Read the model definition and answer for the solid it produces. Units are mm, in the model's axes. A direction names the side the tool comes from. Coordinates: 2 decimals unless noted, no trailing zeros. Write each loop counter-clockwise with the first axis right and the second up, starting at its lowest first coordinate (ties: lowest second). Pieces come first, ordered by that corner, then holes. Notation, with made-up numbers: (-34, 15) -> (-7, 15) arc R14 cw to (-7, 19) -> close; hole circle Ø3 at (49.5, 8.5). An arc over 180 degrees is marked (long way). One line per item, written item: value. Start each with the question number.
1. Consider line 1 along Z through (x, y) = (0, 18); line 2 along X through (y, z) = (-42, 8). Determine where each line is inside the solid, lowest interval first.
2. Find section C-C, the plane x = 0. Write down the section's boundary in (y, z), and give its area (3 significant figures).
3. Find section D-D, the plane x = 24.5. Write down the section's boundary in (y, z).
4. For faces 1 (the flat face through (-30, 5, 20)), 2 (the cylindrical face through (-3.905, 0.7, -29.745)), 3 (the flat face through (63.479, 4.93, 7.606)), 4 (the flat face through (24, 10, 35)), 5 (the flat face through (50, 15, 100)), determine the directions among +Z, -Z, +X, -X, +Y, -Y from which every point of the face is accessible in a straight line to the end or side of a thin tool.
5. Given P1, Ø2, axis at x = 80.5, z = 48, coming from the +Y side; P2, Ø1, axis at x = 49.5, z = 12, coming from the -Y side; P3, Ø10, axis at x = 20.5, y = -11.5, coming from the +Z side, each flat-ended and moving along its own axis, determine where each tip first touches the part or whether it passes through.
6. Find section B-B, the plane z = 84.5. Write down the section's boundary in (x, y), and give its area (3 significant figures).
7. Find section A-A, the plane y = 17.5. Write down the section's boundary in (x, z), and give its area (3 significant figures).
```python
from build123d import *

# Parameters (mm, degrees)
SKETCH1_R                = 30
SKETCH1_R_2              = 15
BOSS_EXTRUDE1_DEPTH      = 10
SKETCH1_3_R              = 30
SKETCH1_3_R_2            = 15
BOSS_EXTRUDE2_DEPTH      = 50
BOSS_EXTRUDE2_DEPTH_BACK = 50
BOSS_EXTRUDE3_DEPTH      = 30


with BuildPart() as part:
    # Sketch1 → Boss-Extrude1 (new body)
    with BuildSketch(Plane(origin=(0, 0, 0), x_dir=(1, 0, 0), z_dir=(0, 1, 0))):
        Circle(SKETCH1_R)
        Circle(SKETCH1_R_2, mode=Mode.SUBTRACT)
        with BuildLine():
            ThreePointArc((30, 0), (0, -30), (-30, 0))
            Line((-30, 0), (-30, -40))
            Line((-30, -40), (44.477364607, -115.187247331))
            ThreePointArc((44.477364607, -115.187247331), (41.7229458, -47.830649341), (108.548527268, -38.951472732))
            Line((108.548527268, -38.951472732), (17.129116361, 24.629116361))
            ThreePointArc((17.129116361, 24.629116361), (26.588282107, 13.894720385), (30, 0))
        make_face()
        with BuildLine():
            Line((110, -80), (110, -120))
            ThreePointArc((110, -120), (80, -30), (50, -120))
            Line((50, -120), (50, -80))
            ThreePointArc((50, -80), (80, -50), (110, -80))
        make_face()
    extrude(amount=BOSS_EXTRUDE1_DEPTH)

    # Sketch1_3 → Boss-Extrude2 (add, two sides)
    with BuildSketch(Plane(origin=(0, 0, 0), x_dir=(1, 0, 0), z_dir=(0, 1, 0))) as boss_extrude2_sk:
        Circle(SKETCH1_3_R)
        Circle(SKETCH1_3_R_2, mode=Mode.SUBTRACT)
    extrude(amount=BOSS_EXTRUDE2_DEPTH)
    extrude(boss_extrude2_sk.sketch, amount=-BOSS_EXTRUDE2_DEPTH_BACK)

    # Sketch1_4 → Boss-Extrude3 (add)
    with BuildSketch(Plane(origin=(0, 0, 0), x_dir=(1, 0, 0), z_dir=(0, 1, 0))):
        with BuildLine():
            Line((110, -80), (110, -120))
            ThreePointArc((110, -120), (80, -30), (50, -120))
            Line((50, -120), (50, -80))
            ThreePointArc((50, -80), (80, -50), (110, -80))
        make_face()
    extrude(amount=BOSS_EXTRUDE3_DEPTH)


solid = part.part
```
Answer block:
1. line 1: z = -30 to -15, 15 to 30
1. line 2: x = -28.91 to -12.69, 12.69 to 28.91
2. outline: (-50, -30) -> (50, -30) -> (50, -15) -> (-50, -15) -> close; (-50, 15) -> (50, 15) -> (50, 30) -> (10, 30) -> (10, 70.29) -> (0, 70.29) -> (0, 30) -> (-50, 30) -> close
2. area: 3,400 mm2
3. outline: (-50, -17.31) -> (0, -17.31) -> (0, -19.5) -> (10, -19.5) -> (10, -17.31) -> (50, -17.31) -> (50, 17.31) -> (10, 17.31) -> (10, 95.02) -> (0, 95.02) -> (0, 17.31) -> (-50, 17.31) -> close
4. face 1: +Z, -Z, -X, +Y, -Y
4. face 2: none
4. face 3: -Z, +X, +Y, -Y
4. face 4: +Y
4. face 5: +Z, +Y, -Y
5. P1: stops at y = 30
5. P2: stops at y = 0
5. P3: stops at z = 25.69
6. outline: (14.08, 0) -> (50, 0) -> (50, 30) -> (30.2, 30) -> (30.2, 10) -> (14.08, 10) -> close; (110, 0) -> (129.8, 0) -> (129.8, 30) -> (110, 30) -> close
6. area: 1,350 mm2
7. outline: circle Ø60 at (0, 0); (50, 80) -> (50, 120) arc R50 ccw (long way) to (110, 120) -> (110, 80) arc R30 cw to start; hole circle Ø30 at (0, 0)
7. area: 5,750 mm2
